```python
from build123d import *

# Parameters (mm, degrees)
BOSS_EXTRUDE1_DEPTH  = 32
M2_CLEARANCE_HOLE1_D = 2.4
FILLET1_R            = 1
SKETCH9_W            = 5.67
SKETCH9_H            = 27
CUT_EXTRUDE1_DEPTH   = 1.5
FILLET2_R            = 1


with BuildPart() as part:
    # Sketch2 → Boss-Extrude1 (new, symmetric)
    with BuildSketch(Plane.XY):
        with BuildLine():
            Line((3.334540069, -5), (-3.334540069, -5))
            ThreePointArc((-3.334540069, -5), (-10.7, -1.5), (-18.065459931, -5))
            Line((-18.065459931, -5), (-21.734540069, -5))
            ThreePointArc((-21.734540069, -5), (-29.1, -1.5), (-36.465459931, -5))
            Line((-36.465459931, -5), (-42.3, -5))
            Line((-42.3, -5), (-42.3, 0))
            Line((-42.3, 0), (42.3, 0))
            Line((42.3, 0), (42.3, -5))
            Line((42.3, -5), (36.465459931, -5))
            ThreePointArc((36.465459931, -5), (29.1, -1.5), (21.734540069, -5))
            Line((21.734540069, -5), (18.065459931, -5))
            ThreePointArc((18.065459931, -5), (10.7, -1.5), (3.334540069, -5))
        make_face()
    extrude(amount=BOSS_EXTRUDE1_DEPTH, both=True)

    # M2 Clearance Hole1 (through all)
    with Locations(Plane(origin=(0, -5, 0), x_dir=(-1, 0, 0), z_dir=(0, -1, 0))):
        with Locations((0, 25), (0, 0), (0, -25), (39.8, -25), (39.8, 0), (39.8, 25), (-39.8, -18), (-39.8, 18)):
            Hole(M2_CLEARANCE_HOLE1_D / 2)

    # Fillet1
    fillet1_edges = [part.edges().sort_by_distance(p)[0] for p in [
        (42.3, -2.5, -32),
        (-42.3, -2.5, -32),
        (-42.3, -2.5, 32),
        (42.3, -2.5, 32),
    ]]
    fillet(fillet1_edges, radius=FILLET1_R)

    # Sketch9 → Cut-Extrude1 (cut)
    with BuildSketch(Plane(origin=(0, 0, 0), x_dir=(1, 0, 0), z_dir=(0, 1, 0))):
        with Locations((39.465, 0)):
            Rectangle(SKETCH9_W, SKETCH9_H)
    extrude(amount=-CUT_EXTRUDE1_DEPTH, mode=Mode.SUBTRACT)

    # Fillet2
    fillet2_edges = [part.edges().sort_by_distance(p)[0] for p in [
        (39.465, -1.5, 13.5),
        (36.63, -1.5, 0),
        (39.465, -1.5, -13.5),
    ]]
    fillet(fillet2_edges, radius=FILLET2_R)


solid = part.part
```
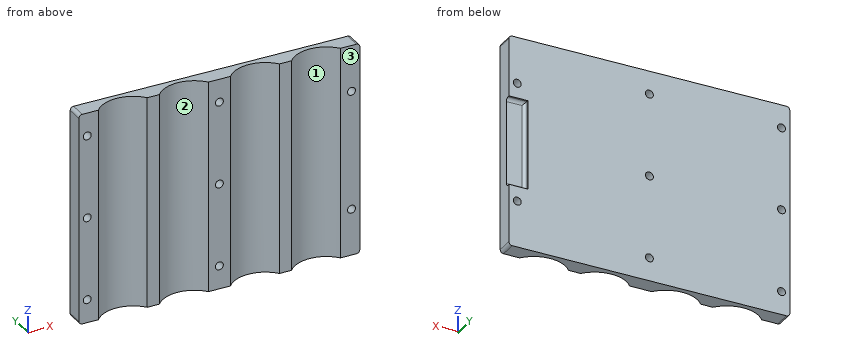
CAD build for the part. Positions are in the model's coordinates, mm. Face numbers are marked on the shaded views. Round coordinates to 2 decimals unless told otherwise and drop trailing zeros. Order: outer loops, then holes, each group sorted by start corner. A loop starts at its lowest first (then second) coordinate and runs counter-clockwise, first axis right, second up. Notation, with made-up numbers: (54.5, 20) -> (104.5, 20) arc R13 ccw to (104.5, 29) -> close; hole circle Ø9 at (83, 82). An arc over 180 degrees is marked (long way). Write item = value, one per line.
(1) Flat gauge pins, fed straight in: P1, Ø2, axis at x = 39.8, z = 18, coming from the +Y side; P2, Ø1.4, axis at x = 40.5, z = -5.5, coming from the +Y side; P3, Ø3, axis at x = 0, z = 25, coming from the +Y side; P4, Ø0.6, axis at y = -0.5, z = 0, coming from the +X side. Where does each tip first touch, or does it go through?
Answers follow:
P1 = through
P2 = -1.5
P3 = 0
P4 = 36.68
(2) Drill centre lines: L1, parallel to Z at x = 0, y = -2.2; L2, parallel to X at y = -1.25, z = -25; L3, parallel to X at y = -2.6, z = 20. Where is each one in solid material? Low to high.
Answers follow:
L1 = -32 to -26.2, -23.8 to -1.2, 1.2 to 23.8, 26.2 to 32
L2 = -42.3 to -41, -38.6 to -1.2, 1.2 to 42.3
L3 = -42.3 to -33.54, -24.66 to -15.14, -6.26 to 6.26, 15.14 to 24.66, 33.54 to 42.3
(3) Cut at D-D (z = 0). Write the cut outline in (x, y).
Answers follow:
outline = (-42.3, -5) -> (-41, -5) -> (-41, 0) -> (-42.3, 0) -> close; (-38.6, -5) -> (-36.47, -5) arc R9.5 cw to (-21.73, -5) -> (-18.07, -5) arc R9.5 cw to (-3.33, -5) -> (-1.2, -5) -> (-1.2, 0) -> (-38.6, 0) -> close; (1.2, -5) -> (3.33, -5) arc R9.5 cw to (18.07, -5) -> (21.73, -5) arc R9.5 cw to (36.47, -5) -> (42.3, -5) -> (42.3, -1.5) -> (37.63, -1.5) arc R1 cw to (36.63, -0.5) -> (36.63, 0) -> (1.2, 0) -> close
(4) Cut at C-C (y = -2.75). State how many separate pieces and enclosed holes the cut face has, plus the area to 3 significant figures.
Answers follow:
separate_pieces = 5
enclosed_holes = 8
area = 2,970 mm²
(5) Cut at B-B (z = -18). Write the cut outline in (x, y), plus the area to 3 significant figures.
Answers follow:
outline = (-42.3, -5) -> (-36.47, -5) arc R9.5 cw to (-21.73, -5) -> (-18.07, -5) arc R9.5 cw to (-3.33, -5) -> (3.33, -5) arc R9.5 cw to (18.07, -5) -> (21.73, -5) arc R9.5 cw to (36.47, -5) -> (38.6, -5) -> (38.6, 0) -> (-42.3, 0) -> close; (41, -5) -> (42.3, -5) -> (42.3, 0) -> (41, 0) -> close
area = 267 mm²
(6) Cut at A-A (x = 39.8). Write the cut outline in (y, z), plus the area to 3 significant figures.
Answers follow:
outline = (-5, -32) -> (0, -32) -> (0, -19.2) -> (-5, -19.2) -> close; (-5, -16.8) -> (0, -16.8) -> (0, -13.5) -> (-0.5, -13.5) arc R1 cw to (-1.5, -12.5) -> (-1.5, 12.5) arc R1 cw to (-0.5, 13.5) -> (0, 13.5) -> (0, 16.8) -> (-5, 16.8) -> close; (-5, 19.2) -> (0, 19.2) -> (0, 32) -> (-5, 32) -> close
area = 256 mm²
(7) Pull direction X, two halves, no side cores. Call the marked faces 1, 2 and 3: +X half, -X half, draft (parallel to the pull), parting line (faces both ways), or undercut.
Answers follow:
face_1 = undercut
face_2 = undercut
face_3 = draft
